Read the model definition and answer for the solid it produces. Units are mm, in the model's axes. A direction names the side the tool comes from. Coordinates: 2 decimals unless noted, no trailing zeros. Loops run counter-clockwise (first coordinate to the right, second up) from the corner with the lowest first, then second, coordinate; pieces in that order, holes last. Notation, with made-up numbers: M 62.25,-34.75 L 101.25,-34.75 A9 cw 101.25,-25.75 Z; hole C 48.5,0 d11. An arc over 180 degrees is marked long. One line per item, written item: value. Start each with the question number.
1. For faces 1 (the face through (0, 64.5, 0)), 2 (the face through (21, 47, -3)), 3 (the face through (-3, 70.5, 0)), determine the directions among +Z, -Z, +X, -X, +Y, -Y from which every point of the face is accessible in a straight line to the end or side of a thin tool.
2. Determine the mould class of faces 4 (the face through (21, 47, 3)), 5 (the face through (7, 74, 0)), 6 (the face through (13, 71, 0)) for opening direction X: +X half, -X half, draft (parallel to the pull), parting line (faces both ways), or undercut.
3. The part is cut by section B-B (z = 8). Write down the section's boundary in (x, y).
4. Consider probe 1 along Y at (x, z) = (-11, 1.7); probe 2 along X at (y, z) = (67.5, 0.5); probe 3 along Y at (x, z) = (-13, 1). Determine where each line is inside the solid, lowest interval first.
5. Flat-ended cylindrical pins translate along their axes: pin 1 (5 mm diameter, centred on x = -11, y = 37.5, fed in from -Z); pin 2 (4 mm diameter, centred on x = 49, z = -11, fed in from +Y); pin 3 (6.5 mm diameter, centred on x = -7, y = 70.5, fed in from -Z); pin 4 (3.5 mm diameter, centred on y = 74, z = -14, fed in from -X). Find the tip coordinate at first contact, or state that the pin passes through.
6. The part is cut by section A-A (x = 57). Write down the section's boundary in (y, z).
```python
from build123d import *

# Parameters (mm, degrees)
BOSS_EXTRU_1_DEPTH      = 75
BOSS_EXTRU_3_DEPTH      = 5
BOSS_EXTRU_3_DEPTH_BACK = 5
ESQUISSE7_R             = 1.5
BOSS_EXTRU_2_DEPTH      = 3
BOSS_EXTRU_2_DEPTH_BACK = 3
ESQUISSE3_R             = 1.5


with BuildPart() as part:
    # Esquisse1 → Boss.-Extru.1 (new body)
    with BuildSketch(Plane(origin=(0, 0, 0), x_dir=(0, 0, -1), z_dir=(1, 0, 0))):
        with BuildLine():
            Line((-37.5, 70.099928673), (-36.556603774, 68.336408455))
            ThreePointArc((-36.556603774, 68.336408455), (0, 77.5), (36.556603774, 68.336408455))
            Line((36.556603774, 68.336408455), (37.5, 70.099928673))
            ThreePointArc((37.5, 70.099928673), (0, 79.5), (-37.5, 70.099928673))
        make_face()
    extrude(amount=BOSS_EXTRU_1_DEPTH)

    # Esquisse7 → Boss.-Extru.3 (add, two sides: drawn at the far end of the back side and taken through both)
    with BuildSketch(Plane.XY.offset(-BOSS_EXTRU_3_DEPTH_BACK)):
        with BuildLine():
            Line((7, 77.5), (7, 70.5))
            Line((7, 70.5), (-13, 70.5))
            ThreePointArc((-13, 70.5), (-16, 67.5), (-13, 64.5))
            Line((-13, 64.5), (13, 64.5))
            Line((13, 64.5), (13, 77.5))
            Line((13, 77.5), (7, 77.5))
        make_face()
        with Locations((-13, 67.5)):
            Circle(ESQUISSE7_R, mode=Mode.SUBTRACT)
    extrude(amount=BOSS_EXTRU_3_DEPTH + BOSS_EXTRU_3_DEPTH_BACK)

    # Esquisse3 → Boss.-Extru.2 (add, two sides: drawn at the far end of the back side and taken through both)
    with BuildSketch(Plane.XY.offset(-BOSS_EXTRU_2_DEPTH_BACK)):
        with BuildLine():
            Line((30.72135955, 77.5), (30.72135955, 72.5))
            add(Edge.make_bspline(
                [(30.72135955, 72.5), (30.72135955, 44.694963761), (24.910353183, 46.831964153), (-11, 40.5)],
                knots=[0, 0, 0, 0, 1, 1, 1, 1], degree=3))
            ThreePointArc((-11, 40.5), (-14, 37.5), (-11, 34.5))
            add(Edge.make_bspline(
                [(36.72135955, 72.5), (36.72135955, 41.406516096), (28.397257564, 41.446799475), (-11, 34.5)],
                knots=[0, 0, 0, 0, 1, 1, 1, 1], degree=3))
            Line((36.72135955, 72.5), (36.72135955, 77.5))
            Line((36.72135955, 77.5), (30.72135955, 77.5))
        make_face()
        with Locations((-11, 37.5)):
            Circle(ESQUISSE3_R, mode=Mode.SUBTRACT)
    extrude(amount=BOSS_EXTRU_2_DEPTH + BOSS_EXTRU_2_DEPTH_BACK)


solid = part.part
```
Answer block:
1. face 1: +Z, -Z, -X
1. face 2: +X, -Y
1. face 3: -X
2. face 4: draft
2. face 5: -X half
2. face 6: undercut
3. outline: M 0,77.09 L 75,77.09 L 75,79.1 L 0,79.1 Z
4. probe 1: y = 34.5 to 36, 39 to 40.5, 64.5 to 70.5
4. probe 2: x = -16 to -14.5, -11.5 to 13, 30.64 to 36.64
4. probe 3: y = 35.26 to 39.74, 64.5 to 66, 69 to 70.5
5. pin 1: stops at z = -3
5. pin 2: stops at y = 78.99
5. pin 3: stops at z = -5
5. pin 4: passes through
6. outline: M 68.34,-36.56 L 70.1,-37.5 A79.5 ccw 70.1,37.5 L 68.34,36.56 A77.5 cw Z
